CAD build for the part. Positions are in the model's coordinates, mm. Face numbers are marked on the shaded views. A direction names the side the tool comes from. Coordinates: 2 decimals unless noted, no trailing zeros. Write each loop counter-clockwise with the first axis right and the second up, starting at its lowest first coordinate (ties: lowest second). Pieces come first, ordered by that corner, then holes. Notation, with made-up numbers: (67.5, -35.75) - (85.5, -35.75) arc R25 ccw to (85.5, -1.75) - close; hole circle Ø10 at (-11.75, 7.5). An arc over 180 degrees is marked (long way). One line per question, with ' | ' between items. Start each with the question number.
1. Probe line 1 (X direction, y = 1.9, z = 12.5); line 2 (Z direction, x = -14.5, y = 0.5); line 3 (X direction, y = 4.5, z = -2) (3 decimals). List the from-to ranges inside material, lowest first.
2. Band-saw the part on C-C, the plane x = -10. Write the cut outline in (y, z).
3. Band-saw the part on A-A, the plane z = 3.5. Write the cut outline in (x, y).
4. Band-saw the part on D-D, the plane x = 10. Write the cut outline in (y, z).
5. Band-saw the part on B-B, the plane z = -12.5. Write the cut outline in (x, y).
6. Which spindle directions (+Z, -Z, +X, -X, +Y, -Y) get a long thin tool onto all of the face, cutting with end or side? Do the marked faces 1, 2 and 3. Say none if no direction does.
7. Two-plate mould, pull along Z, no slides. Class the marked faces 4, 5, 6 and 7: +Z half, -Z half, draft (parallel to the pull), parting line (faces both ways), or undercut.
8. Flat gauge pins, fed straight in: P1, Ø5, axis at x = -17, z = -12.5, coming from the +Y side; P2, Ø3.5, axis at x = 1.5, y = 8, coming from the -Z side; P3, Ø1, axis at x = -4.5, z = 9, coming from the +Y side. Where does each tip first touch, or does it go through?
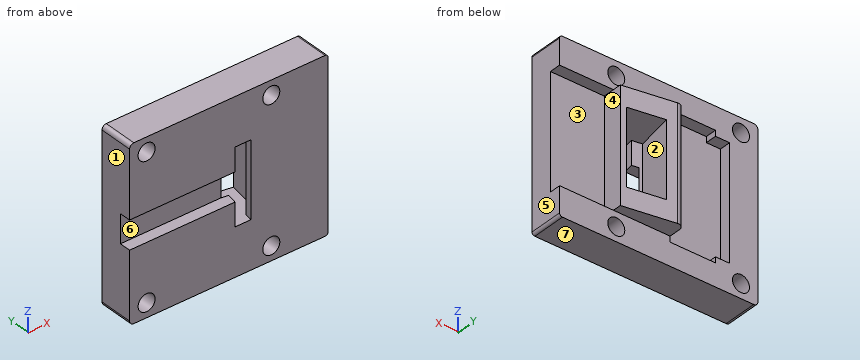
from build123d import *

# Parameters (mm, degrees)
SKETCH1_W                = 30
SKETCH1_H                = 20
BASE_PLATE_DEPTH         = 1
SIDE_WALLS_DEPTH         = 6
SKETCH3_W                = 10
SKETCH3_H                = 20
SWITCH_BLOCK_DEPTH       = 6.5
SKETCH11_W               = 10.5
SKETCH11_H               = 20
SKETCH11_W_2             = 9.5
THICKER_BODY_DEPTH       = 3
SWITCH_BLOCK_ANGLE_DEPTH = 20
SKETCH4_R                = 1.5
M2_SCREWS_DEPTH          = 6
FILLET1_R                = 1
FILLET2_R                = 0.5
FILLET3_R                = 0.5
FILLET4_R                = 0.75
FILLET5_R                = 0.75
SKETCH19_W               = 8
SKETCH19_H               = 22
SPACE_FOR_LEAVER_DEPTH   = 2
SKETCH22_W               = 6.25
SKETCH22_H               = 13.25
SWITCH_DEPTH             = 6.75
SKETCH23_W               = 2.75
SKETCH23_H               = 13.25
CUT_EXTRUDE2_DEPTH       = 27.310171552
SKETCH24_W               = 20
SKETCH24_H               = 5
CUT_EXTRUDE3_DEPTH       = 2


with BuildPart() as part:
    # Sketch1 → Base Plate (new body)
    with BuildSketch(Plane(origin=(0, 0, 0), x_dir=(1, 0, 0), z_dir=(0, 1, 0))):
        Rectangle(SKETCH1_W, SKETCH1_H)
    extrude(amount=BASE_PLATE_DEPTH)

    # Sketch2 → Side Walls (add)
    with BuildSketch(Plane.XZ):
        Polygon((15, 10), (-15, 10), (-15, -10), (15, -10), (15, -15), (-20, -15), (-20, 15), (15, 15), align=None)
    extrude(amount=-SIDE_WALLS_DEPTH)

    # Sketch3 → Switch Block (add)
    with BuildSketch(Plane(origin=(0, 1, 0), x_dir=(1, 0, 0), z_dir=(0, 1, 0))):
        with Locations((0.5, 0)):
            Rectangle(SKETCH3_W, SKETCH3_H)
    extrude(amount=SWITCH_BLOCK_DEPTH)

    # Sketch11 → Thicker Body (add)
    with BuildSketch(Plane(origin=(0, 1, 0), x_dir=(1, 0, 0), z_dir=(0, 1, 0))):
        with Locations((-9.75, 0)):
            Rectangle(SKETCH11_W, SKETCH11_H)
        with Locations((10.25, 0)):
            Rectangle(SKETCH11_W_2, SKETCH11_H)
    extrude(amount=THICKER_BODY_DEPTH)

    # Sketch5 → Switch Block Angle (add)
    with BuildSketch(Plane(origin=(0, 0, -10), x_dir=(-1, 0, 0), z_dir=(0, 0, -1))):
        Polygon((4.5, 7.5), (4.5, 9.25), (-5.5, 7.5), align=None)
    extrude(amount=-SWITCH_BLOCK_ANGLE_DEPTH)

    # Sketch4 → M2 Screws (cut)
    with BuildSketch(Plane(origin=(0, 6, 0), x_dir=(1, 0, 0), z_dir=(0, 1, 0))):
        with Locations(Location((-17, -12.5, 0), (0, 0, 270))):
            Circle(SKETCH4_R)
        with Locations(Location((5, -12.5, 0), (0, 0, 270))):
            Circle(SKETCH4_R)
        with Locations(Location((5, 12.5, 0), (0, 0, 270))):
            Circle(SKETCH4_R)
        with Locations(Location((-17, 12.5, 0), (0, 0, 270))):
            Circle(SKETCH4_R)
    extrude(amount=-M2_SCREWS_DEPTH, mode=Mode.SUBTRACT)

    # Fillet1
    fillet1_edges = [part.edges().sort_by_distance(p)[0] for p in [
        (-4.5, 9.25, 0),
    ]]
    fillet(fillet1_edges, radius=FILLET1_R)

    # Fillet2
    fillet2_edges = [part.edges().sort_by_distance(p)[0] for p in [
        (15, 3, 15),
    ]]
    fillet(fillet2_edges, radius=FILLET2_R)

    # Fillet3
    fillet3_edges = [part.edges().sort_by_distance(p)[0] for p in [
        (15, 3, -15),
    ]]
    fillet(fillet3_edges, radius=FILLET3_R)

    # Fillet4
    fillet4_edges = [part.edges().sort_by_distance(p)[0] for p in [
        (-20, 3, -15),
    ]]
    fillet(fillet4_edges, radius=FILLET4_R)

    # Fillet5
    fillet5_edges = [part.edges().sort_by_distance(p)[0] for p in [
        (-20, 3, 15),
    ]]
    fillet(fillet5_edges, radius=FILLET5_R)

    # Sketch19 → Space for LEaver (cut)
    with BuildSketch(Plane(origin=(0, 6, 0), x_dir=(1, 0, 0), z_dir=(0, 1, 0))):
        with Locations((-8.5, 0)):
            Rectangle(SKETCH19_W, SKETCH19_H)
    extrude(amount=-SPACE_FOR_LEAVER_DEPTH, mode=Mode.SUBTRACT)

    # Sketch22 → Switch (cut)
    with BuildSketch(Plane(origin=(1.436931474, 8.211036992, 0), x_dir=(0.9850304671557042, -0.1723803317522482, 0), z_dir=(0.1723803317522482, 0.9850304671557042, 0))):
        Rectangle(SKETCH22_W, SKETCH22_H)
    extrude(amount=-SWITCH_DEPTH, mode=Mode.SUBTRACT)

    # Sketch23 → Cut-Extrude2 (cut, through all)
    with BuildSketch(Plane(origin=(0.273364234, 1.562081339, 0), x_dir=(0.9850304671557042, -0.1723803317522482, 0), z_dir=(0.1723803317522482, 0.9850304671557042, 0))):
        Rectangle(SKETCH23_W, SKETCH23_H)
    extrude(amount=-CUT_EXTRUDE2_DEPTH, mode=Mode.SUBTRACT)

    # Sketch24 → Cut-Extrude3 (cut)
    with BuildSketch(Plane.XZ):
        with Locations((-10, 0)):
            Rectangle(SKETCH24_W, SKETCH24_H)
    extrude(amount=-CUT_EXTRUDE3_DEPTH, mode=Mode.SUBTRACT)


solid = part.part
Filled in:
1) line 1: x = -20 to -18.5, -15.5 to 3.5, 6.5 to 15 | line 2: z = -15 to -2.5, 2.5 to 15 | line 3: x = -20 to -15, -4.5 to -2.385, 3.96 to 5.5
2) outline: (0, -15) - (6, -15) - (6, -11) - (4, -11) - (4, 11) - (6, 11) - (6, 15) - (0, 15) - (0, 2.5) - (2, 2.5) - (2, -2.5) - (0, -2.5) - close
3) outline: (-20, 0) - (-1.4, 0) - (-1.08, 1.8) - (-2.8, 2.1) - (-1.64, 8.75) - (-3.33, 9.04) arc R1 ccw to (-4.5, 8.06) - (-4.5, 4) - (-15, 4) - (-15, 6) - (-20, 6) - close; (1.4, 0) - (15, 0) - (15, 4) - (5.5, 4) - (5.5, 7.5) - (4.52, 7.67) - (3.35, 1.02) - (1.63, 1.33) - close
4) outline: (0, -15) - (6, -15) - (6, -10) - (4, -10) - (4, 10) - (6, 10) - (6, 15) - (0, 15) - close
5) outline: (-20, 0) - (-18.5, 0) - (-18.5, 6) - (-20, 6) - close; (-15.5, 0) - (3.5, 0) - (3.5, 6) - (-15.5, 6) - close; (6.5, 0) - (15, 0) - (15, 6) - (6.5, 6) - close
6) face 1: +Z, -Z, -X, +Y, -Y | face 2: none | face 3: +X, +Y
7) face 4: undercut | face 5: draft | face 6: undercut | face 7: -Z half
8) P1: stops at y = 6 | P2: stops at z = -10 | P3: stops at y = 8.93
